```python
from build123d import *

# Parameters (mm, degrees)
ESBO_O1_W                = 35
ESBO_O1_H                = 20
RESSALTO_EXTRUS_O1_DEPTH = 10
ESBO_O2_W                = 10
ESBO_O2_H                = 13
RESSALTO_EXTRUS_O2_DEPTH = 5
ESBO_O3_R                = 0.922121428
ESBO_O3_R_2              = 0.963466347
RESSALTO_EXTRUS_O3_DEPTH = 5


with BuildPart() as part:
    # Esboço1 → Ressalto-extrusão1 (new body)
    with BuildSketch(Plane.XY):
        with Locations((1.225709868, 0.66677589)):
            Rectangle(ESBO_O1_W, ESBO_O1_H)
    extrude(amount=RESSALTO_EXTRUS_O1_DEPTH)

    # Esboço2 → Ressalto-extrusão2 (add)
    with BuildSketch(Plane.XY.offset(10)):
        with Locations((-11.274290132, -2.83322411)):
            Rectangle(ESBO_O2_W, ESBO_O2_H)
    extrude(amount=RESSALTO_EXTRUS_O2_DEPTH)

    # Esboço3 → Ressalto-extrusão3 (add)
    with BuildSketch(Plane(origin=(18.725709868, 0, 0), x_dir=(0, 0, -1), z_dir=(1, 0, 0))):
        with Locations((-5.13508621, -6.301169804)):
            Circle(ESBO_O3_R)
        with Locations((-5.13508621, 7.750286856)):
            Circle(ESBO_O3_R_2)
    extrude(amount=RESSALTO_EXTRUS_O3_DEPTH)


solid = part.part
```
Model file for the job. Use its own axes, mm. Round coordinates to 2 decimals unless told otherwise and drop trailing zeros. Order: outer loops, then holes, each group sorted by start corner. A loop starts at its lowest first (then second) coordinate and runs counter-clockwise, first axis right, second up. Notation, with made-up numbers: (80, -33.75) -> (99, -33.75) arc R8 ccw to (99, -21.75) -> close; hole circle Ø4 at (38, 13.5). An arc over 180 degrees is marked (long way). Use one line per item in the form item = value.
Item 1: Pull direction Y, two halves, no side cores. Call faces 1 (the face through (21.2, 6.8, 5.3)), 2 (the face through (21.191, -5.524, 4.639)), 3 (the face through (-11, 3.667, 12)), 4 (the face through (-6.274, -3, 12)): released by +Y, released by -Y, zero draft, split by the parting line, or undercut.
Returned:
face_1 = undercut
face_2 = undercut
face_3 = released by +Y
face_4 = zero draft
Item 2: Cut at D-D, the plane x = -10. Write the cut outline in (y, z), and give its area (3 significant figures).
Returned:
outline = (-9.33, 0) -> (10.67, 0) -> (10.67, 10) -> (3.67, 10) -> (3.67, 15) -> (-9.33, 15) -> close
area = 265 mm^2
Item 3: Cut at A-A, the plane y = -4.5. Write the cut outline in (x, z), and give its area (3 significant figures).
Returned:
outline = (-16.27, 0) -> (18.73, 0) -> (18.73, 10) -> (-6.27, 10) -> (-6.27, 15) -> (-16.27, 15) -> close
area = 400 mm^2
Item 4: Cut at C-C, the plane x = -5. Write the cut outline in (y, z), and give its area (3 significant figures).
Returned:
outline = (-9.33, 0) -> (10.67, 0) -> (10.67, 10) -> (-9.33, 10) -> close
area = 200 mm^2
Item 5: Cut at B-B, the plane z = 5.25. Write the cut outline in (x, y), and give its area (3 significant figures).
Returned:
outline = (-16.27, -9.33) -> (18.73, -9.33) -> (18.73, -7.22) -> (23.73, -7.22) -> (23.73, -5.39) -> (18.73, -5.39) -> (18.73, 6.79) -> (23.73, 6.79) -> (23.73, 8.71) -> (18.73, 8.71) -> (18.73, 10.67) -> (-16.27, 10.67) -> close
area = 719 mm^2
Item 6: Flat gauge pins, fed straight in: pin 1 Ø1 at (x, y) = (14, -1.5) entering from +Z; pin 2 Ø4 at (y, z) = (0, 11.5) entering from +X; pin 3 Ø5.5 at (x, z) = (-12, 13.5) entering from +Y; pin 4 Ø5 at (x, z) = (4, 13) entering from +Y. Where does each tip first touch, or does it go through?
Returned:
pin_1 = 10
pin_2 = 18.73
pin_3 = 3.67
pin_4 = through
Item 7: Drill centre lines: line 1 (X direction, y = 3.5, z = 13); line 2 (Z direction, x = -4, y = 1.5); line 3 (X direction, y = 4.75, z = 4). Where is each one in solid material? Low to high.
Returned:
line_1 = -16.27 to -6.27
line_2 = 0 to 10
line_3 = -16.27 to 18.73
